The model under review builds one solid part; all positions refer to its coordinate system, in mm. Give positions to 0.01 mm unless a question says otherwise; leave off trailing zeros. Write each loop counter-clockwise with the first axis right and the second up, starting at its lowest first coordinate (ties: lowest second). Pieces come first, ordered by that corner, then holes.
from build123d import *

# Parameters (mm, degrees)
SKETCH2_R           = 10.530885837
SKETCH2_R_2         = 6.35
SKETCH3_R           = 10.530885837
SKETCH3_R_2         = 6.35
BOSS_EXTRUDE1_DEPTH = 76.2
SKETCH4_R           = 10.530885837
SKETCH4_R_2         = 6.35
BOSS_EXTRUDE2_DEPTH = 25.4


with BuildPart() as part:
    # Sweep1: sweep along a path in Sketch1
    with BuildLine(Plane(origin=(0, 0, 0), x_dir=(1, 0, 0), z_dir=(0, 1, 0))) as sweep1_path:
        ThreePointArc((0, 0), (-22.86803443, 9.472250006), (-32.340284436, 32.340284436))
    # Sketch2 → Sweep1 (sweep)
    with BuildSketch(Plane(origin=(0, 0, 0), x_dir=(0, 0, -1), z_dir=(1, 0, 0))):
        Circle(SKETCH2_R)
        Circle(SKETCH2_R_2, mode=Mode.SUBTRACT)
    sweep(path=sweep1_path.line)

    # Sketch3 → Boss-Extrude1 (add)
    with BuildSketch(Plane(origin=(0, 0, -32.340284436), x_dir=(-1, 0, 0), z_dir=(0, 0, -1))):
        with Locations((32.340284436, 0)):
            Circle(SKETCH3_R)
        with Locations((32.340284436, 0)):
            Circle(SKETCH3_R_2, mode=Mode.SUBTRACT)
    extrude(amount=BOSS_EXTRUDE1_DEPTH)

    # Sketch4 → Boss-Extrude2 (add)
    with BuildSketch(Plane(origin=(0, 0, 0), x_dir=(0, 0, -1), z_dir=(1, 0, 0))):
        with Locations(Location((0, 0, 0), (0, 0, 180))):
            Circle(SKETCH4_R)
        with Locations(Location((0, 0, 0), (0, 0, 180))):
            Circle(SKETCH4_R_2, mode=Mode.SUBTRACT)
    extrude(amount=BOSS_EXTRUDE2_DEPTH)


solid = part.part
1) To check wall thickness, follow probe 1 along Y at (x, z) = (14, 0); probe 2 along X at (y, z) = (2.25, -73); probe 3 along Z at (x, y) = (-17, -5.5). State the ranges of each line that lie inside material, in increasing order.
2) Consider section C-C, the plane x = 11. Give the boundary of the cut face in (y, z).
3) The part is to be moulded in two halves that separate along Z. For faces 1 (the flat face through (-37, -5, -108.54)), 2 (the cylindrical face through (12.522, 5.634, 2.93)), 3 (the cylindrical face through (12.522, -3.163, 10.045)), 4 (the flat face through (25.4, 5, 5)), say which applies: +Z half, -Z half, draft (parallel to the pull), parting line (faces both ways), or undercut.
4) Consider section B-B, the plane z = -76. Give the boundary of the cut face in (x, y), then the cut area to 3 significant figures.
5) Insertion check: pin 1 (1 mm diameter, centred on y = 7, z = -84.5, fed in from +X); pin 2 (12 mm diameter, centred on y = -8, z = -74, fed in from +X); pin 3 (10 mm diameter, centred on y = 8, z = -22, fed in from -X). Each pin has a flat end and moves straight along its axis. Give the tip position at first contact, or say it passes through.
6) Consider section D-D, the plane y = 8.25. Give the boundary of the cut face in (x, z) (3 decimals), then the cut area to 3 significant figures.
7) Consider section A-A, the plane y = 0. Give the boundary of the cut face in (x, z).
Answer block:
1. probe 1: y = -10.53 to -6.35, 6.35 to 10.53
1. probe 2: x = -42.63 to -38.28, -26.4 to -22.05
1. probe 3: z = -16.32 to -8.64, -1.16 to 5.32
2. outline: circle Ø21.06 at (0, 0); hole circle Ø12.7 at (0, 0)
3. face 1: -Z half
3. face 2: undercut
3. face 3: parting line
3. face 4: draft
4. outline: circle Ø21.06 at (-32.34, 0); hole circle Ø12.7 at (-32.34, 0)
4. area: 222 mm2
5. pin 1: stops at x = -24.05
5. pin 2: stops at x = -22
5. pin 3: stops at x = -41.48
6. outline: (-38.885, -108.54) - (-25.795, -108.54) - (-25.795, -32.34) arc R25.795 cw to (0, -6.545) - (25.4, -6.545) - (25.4, 6.545) - (0, 6.545) arc R38.885 ccw to (-38.885, -32.34) - close
6. area: 1,990 mm2
7. outline: (-42.87, -108.54) - (-38.69, -108.54) - (-38.69, -32.34) arc R38.69 cw to (0, 6.35) - (25.4, 6.35) - (25.4, 10.53) - (0, 10.53) arc R42.87 ccw to (-42.87, -32.34) - close; (-25.99, -108.54) - (-21.81, -108.54) - (-21.81, -32.34) arc R21.81 cw to (0, -10.53) - (25.4, -10.53) - (25.4, -6.35) - (0, -6.35) arc R25.99 ccw to (-25.99, -32.34) - close
